Source: CAD feature listing. Evaluate the final solid. Frame: model axes, mm. Face numbers are marked on the shaded views. A direction names the side the tool comes from. Coordinates: 2 decimals unless noted, no trailing zeros. Write each loop counter-clockwise with the first axis right and the second up, starting at its lowest first coordinate (ties: lowest second). Pieces come first, ordered by that corner, then holes. Notation, with made-up numbers: M 65,19 L 85,19 A28 ccw 85,38 Z; hole C -37.75,24 d8. An arc over 180 degrees is marked long. Write item = value, one per line. Start each with the question number.
1. Section query D-D (z = 11). Output: boundary loops of the cut face in (x, y).
2. Section query B-B (z = 7.25). Output: boundary loops of the cut face in (x, y).
3. Section query A-A (y = 0). Output: boundary loops of the cut face in (x, z).
4. Pull-direction query (X, two-part tool) for the marked faces 3, 4, 5 and 6; classes: pulls with the +X half, pulls with the -X half, needs draft (parallel to the pull), parting line crosses it, or undercut.
5. Pin query (flat end, axial travel): pin 1 Ø6 at (x, z) = (22, 8) entering from +Y; pin 2 Ø5 at (y, z) = (14.5, 7.5) entering from +X; pin 3 Ø6.5 at (x, z) = (-26.25, 10) entering from +Y; pin 4 Ø2.5 at (x, z) = (26.25, 10) entering from +Y. Return the tip coordinate at first contact, or that it passes through.
6. Section query C-C (x = -26.25). Output: boundary loops of the cut face in (y, z).
7. Line query: line 1 along Z through (x, y) = (-26.25, -27.25); line 2 along Y through (x, z) = (-18, 1); line 3 along Y through (x, z) = (11.5, 16.5). Output: solid intervals per line, ascending.
8. Access query for the marked faces 1 and 2. Directions: +Z, -Z, +X, -X, +Y, -Y. A direction counts if a zero-diameter tool reaches every point of the face in a straight line with its end or side. Return the directions, or none.
```python
from build123d import *

# Parameters (mm, degrees)
SKETCH1_R           = 22.5
SKETCH1_R_2         = 20.5
BOSS_EXTRUDE2_DEPTH = 20
SKETCH2_W           = 60
SKETCH2_H           = 10
BOSS_EXTRUDE3_DEPTH = 20
SKETCH3_R           = 2
CUT_EXTRUDE1_DEPTH  = 20


with BuildPart() as part:
    # Sketch1 → Boss-Extrude2 (new body)
    with BuildSketch(Plane.XY):
        Circle(SKETCH1_R)
        Circle(SKETCH1_R_2, mode=Mode.SUBTRACT)
    extrude(amount=BOSS_EXTRUDE2_DEPTH)

    # Sketch2 → Boss-Extrude3 (add)
    with BuildSketch(Plane(origin=(0, 0, 0), x_dir=(-1, 0, 0), z_dir=(0, 0, -1))):
        with Locations((0, -25.5)):
            Rectangle(SKETCH2_W, SKETCH2_H)
    extrude(amount=-BOSS_EXTRUDE3_DEPTH)

    # Sketch3 → Cut-Extrude1 (cut)
    with BuildSketch(Plane(origin=(0, -20.5, 0), x_dir=(1, 0, 0), z_dir=(0, 1, 0))):
        with Locations(Location((26.25, -10, 0), (0, 0, 180))):
            Circle(SKETCH3_R)
        with Locations(Location((-26.25, -10, 0), (0, 0, 180))):
            Circle(SKETCH3_R)
    extrude(amount=-CUT_EXTRUDE1_DEPTH, mode=Mode.SUBTRACT)


solid = part.part
```
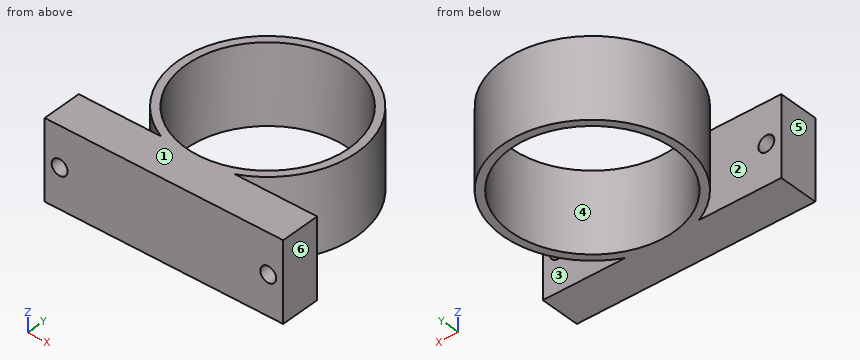
Results are:
q1.outline = M -30,-30.5 L -27.98,-30.5 L -27.98,-20.5 L -30,-20.5 Z; M -24.52,-30.5 L 24.52,-30.5 L 24.52,-20.5 L 9.27,-20.5 A22.5 ccw long -9.27,-20.5 L -24.52,-20.5 Z; M 27.98,-30.5 L 30,-30.5 L 30,-20.5 L 27.98,-20.5 Z; hole C 0,0 d41
q2.outline = M -30,-30.5 L 30,-30.5 L 30,-20.5 L 9.27,-20.5 A22.5 ccw long -9.27,-20.5 L -30,-20.5 Z; hole C 0,0 d41
q3.outline = M -22.5,0 L -20.5,0 L -20.5,20 L -22.5,20 Z; M 20.5,0 L 22.5,0 L 22.5,20 L 20.5,20 Z
q4.face_3 = needs draft
q4.face_4 = undercut
q4.face_5 = pulls with the -X half
q4.face_6 = pulls with the +X half
q5.pin_1 = 12.05
q5.pin_2 = 19.03
q5.pin_3 = -20.5
q5.pin_4 = through
q6.outline = M -30.5,0 L -20.5,0 L -20.5,8 L -30.5,8 Z; M -30.5,12 L -20.5,12 L -20.5,20 L -30.5,20 Z
q7.line_1 = 0 to 8, 12 to 20
q7.line_2 = -30.5 to -20.5, -13.5 to -9.81, 9.81 to 13.5
q7.line_3 = -30.5 to -20.5, -19.34 to -16.97, 16.97 to 19.34
q8.face_1 = +Z, +X, -X, +Y, -Y
q8.face_2 = +Z, -Z, -X
